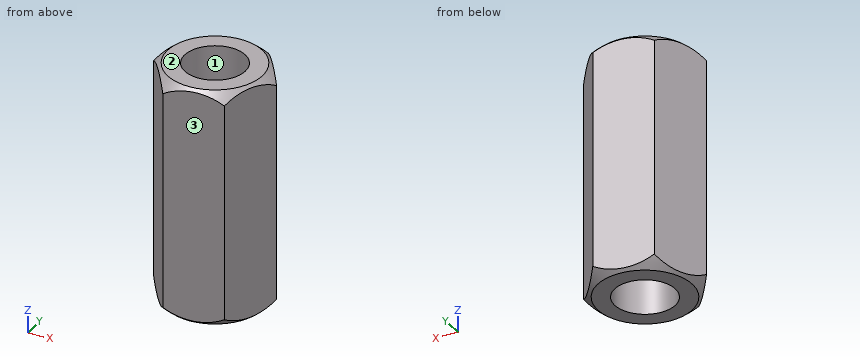
```python
from build123d import *

# Parameters (mm, degrees)
EXTRUSION1_DEPTH   = 40
TROU_TARAUD_M121_D = 10.2


with BuildPart() as part:
    # Esquisse1 → Extrusion1 (new body)
    with BuildSketch(Plane.XY):
        Polygon((3.813132395, 9.043967861), (-5.925739721, 7.824253453), (-9.738872116, -1.219714408), (-3.813132395, -9.043967861), (5.925739721, -7.824253453), (9.738872116, 1.219714408), align=None)
    extrude(amount=EXTRUSION1_DEPTH)

    # Trou taraudé M121 (through all)
    with Locations(Plane(origin=(0, 0, 0), x_dir=(-1, 0, 0), z_dir=(0, 0, -1))):
        with Locations((0, 0)):
            Hole(TROU_TARAUD_M121_D / 2)

    # Esquisse5 → Enlèvement de matière-Révolution1 (revolve, cut)
    with BuildSketch(Plane(origin=(0, 0, 0), x_dir=(1, 0, 0), z_dir=(0, 1, 0)), mode=Mode.PRIVATE) as enl_vement_de_mati_re_r_volution1_sk:
        with BuildLine():
            Line((0, 7.38932546), (0, 2.731180457))
            ThreePointArc((0, 2.731180457), (9.188017929, -1.07462118), (12.993819567, -10.26263911))
            Line((12.993819567, -10.26263911), (12.993819567, 7.38932546))
            Line((12.993819567, 7.38932546), (0, 7.38932546))
        make_face()
        with BuildLine():
            Line((12.993819567, -47.38932546), (12.993819567, -29.73736089))
            ThreePointArc((12.993819567, -29.73736089), (9.188017929, -38.92537882), (0, -42.731180457))
            Line((0, -42.731180457), (0, -47.38932546))
            Line((0, -47.38932546), (12.993819567, -47.38932546))
        make_face()
    revolve(enl_vement_de_mati_re_r_volution1_sk.sketch.rotate(Axis((0, 0, 10.26263911), (0, 0, -1)), 352.861339984), axis=Axis((0, 0, 10.26263911), (0, 0, -1)), mode=Mode.SUBTRACT)


solid = part.part
```
Here's how the part is built. I have some questions about the finished solid (model axes, mm). Face numbers are marked on the shaded views. Coordinates: 2 decimals unless noted, no trailing zeros. Loops run counter-clockwise (first coordinate to the right, second up) from the corner with the lowest first, then second, coordinate; pieces in that order, holes last. Notation, with made-up numbers: (-33.5, 61) -> (-2.5, 61) arc R30 ccw to (-2.5, 92) -> close; hole circle Ø5 at (-28, -7.75). An arc over 180 degrees is marked (long way). Return JSON: item names as keys, results as strings.
1) If we section it at D-D, the plane x = -6.75: Write out the boundary of the cut face in (y, z), then the cut area to 3 significant figures.
Results below:
{"outline": "(-5.17, 0.43) arc R11.1 ccw to (-4.24, 0) -> (4.24, 0) arc R11.1 ccw to (5.87, 0.84) -> (5.87, 39.16) arc R11.1 ccw to (4.24, 40) -> (-4.24, 40) arc R11.1 ccw to (-5.17, 39.57) -> close", "area": "440 mm²"}
2) If we section it at C-C, the plane x = 0: Write out the boundary of the cut face in (y, z).
Results below:
{"outline": "(-8.57, 0.49) arc R12.99 ccw to (-7.97, 0) -> (-5.1, 0) -> (-5.1, 40) -> (-7.97, 40) arc R12.99 ccw to (-8.57, 39.51) -> close; (5.1, 0) -> (7.97, 0) arc R12.99 ccw to (8.57, 0.49) -> (8.57, 39.51) arc R12.99 ccw to (7.97, 40) -> (5.1, 40) -> close"}
3) Thinking about a two-plate mould opening in Y: for the marked faces 1, 2 and 3, which applies, +Y half, -Y half, draft (parallel to the pull), parting line (faces both ways), or undercut?
Results below:
{"face 1": "undercut", "face 2": "draft", "face 3": "-Y half"}
4) If we section it at A-A, the plane z = 24: Write out the boundary of the cut face in (x, y).
Results below:
{"outline": "(-9.74, -1.22) -> (-3.81, -9.04) -> (5.93, -7.82) -> (9.74, 1.22) -> (3.81, 9.04) -> (-5.93, 7.82) -> close; hole circle Ø10.2 at (0, 0)"}
5) I need wall thicknesses on line 1 (X direction, y = -3.25, z = 21.5); line 2 (X direction, y = -0.5, z = 36); line 3 (Y direction, x = 2, z = 32). Which ranges of each line are inside material? Lowest first, please. Write a range as from..to.
Results below:
{"line 1": "-8.2..-3.93, 3.93..7.85", "line 2": "-9.44..-5.08, 5.08..9.01", "line 3": "-8.32..-4.69, 4.69..8.82"}
6) Will these pins go through, and if not, where does the flat tip stop? pin 1 (10 mm diameter, centred on y = 0, z = 29.5, fed in from -X); pin 2 (2 mm diameter, centred on x = -3, z = 17.5, fed in from +Y); pin 3 (8 mm diameter, centred on y = 5, z = 21.5, fed in from +X); pin 4 (10 mm diameter, centred on x = -2, z = 31, fed in from -Y).
Results below:
{"pin 1": "x = -9.74", "pin 2": "y = 8.32", "pin 3": "x = 9.74", "pin 4": "y = -9.04"}
7) If we section it at B-B, the plane y = -0.5: Write out the boundary of the cut face in (x, z).
Results below:
{"outline": "(-9.44, 1.34) arc R12.98 ccw to (-7.95, 0) -> (-5.08, 0) -> (-5.08, 40) -> (-7.95, 40) arc R12.98 ccw to (-9.44, 38.66) -> close; (5.08, 0) -> (7.95, 0) arc R12.98 ccw to (9.01, 0.92) -> (9.01, 39.08) arc R12.98 ccw to (7.95, 40) -> (5.08, 40) -> close"}
